```python
from build123d import *

# Parameters (mm, degrees)
BOSS_EXTRUDE1_DEPTH = 3.175
BOSS_EXTRUDE3_DEPTH = 152.4
BOSS_EXTRUDE4_DEPTH = 3.175
FILLET1_R           = 3.175
CHAMFER1_SIZE2      = 11.849261314
CHAMFER1_SIZE       = 3.175
SKETCH4_R           = 1.905
CUT_EXTRUDE1_DEPTH  = 158.75
CUT_EXTRUDE2_DEPTH  = 254


# Some blends are built 0.0001 mm under size
with BuildPart() as part:
    # Sketch1 → Boss-Extrude1 (new body)
    with BuildSketch(Plane(origin=(0, 0, 0), x_dir=(1, 0, 0), z_dir=(0, 1, 0))):
        Polygon((0, 0), (76.2, 0), (76.2, 63.5), (-17.014773719, 63.5), align=None)
    extrude(amount=BOSS_EXTRUDE1_DEPTH)

    # Sketch2 → Boss-Extrude3 (add)
    with BuildSketch(Plane(origin=(0, 3.175, 0), x_dir=(1, 0, 0), z_dir=(0, 1, 0))):
        Polygon((76.2, 0), (0, 0), (-17.014773719, 63.5), (-13.727771847, 63.5), (2.436263187, 3.175), (76.2, 3.175), align=None)
    extrude(amount=BOSS_EXTRUDE3_DEPTH)

    # Sketch3 → Boss-Extrude4 (add)
    with BuildSketch(Plane(origin=(0, 155.575, 0), x_dir=(1, 0, 0), z_dir=(0, 1, 0))):
        Polygon((-17.014773719, 63.5), (0, 0), (76.2, 0), (76.2, 63.5), align=None)
    extrude(amount=BOSS_EXTRUDE4_DEPTH)

    # Fillet1
    # the kernel refuses this fillet: 3.175 mm, written as the material it takes off along each edge
    with BuildSketch(Plane(origin=(2.436263187, 3.175, -3.175), x_dir=(-0.9659258262890689, 0, 0.2588190451025188), z_dir=(0, -1, 0))) as fillet1_piece_1_section:
        Polygon((0, 0), (FILLET1_R * 1.02, 0), (FILLET1_R * 1.02, -FILLET1_R * 0.782673527739), (FILLET1_R * 0.263995426005, -FILLET1_R * 0.985244342815), align=None)
    fillet1_piece_1 = extrude(amount=FILLET1_R * 1.02, mode=Mode.PRIVATE)
    fillet1_piece_1 = fillet1_piece_1 - Plane(origin=(2.436263187, 3.175, -3.175), x_dir=(0.6087614290087213, 0, -0.7933533402912346), z_dir=(0, -1, 0)) * Sphere(FILLET1_R, mode=Mode.PRIVATE)
    add(fillet1_piece_1, mode=Mode.SUBTRACT)
    with BuildSketch(Plane(origin=(2.436263187, 155.575, -3.175), x_dir=(0, 0, 1), z_dir=(0, 1, 0))) as fillet1_piece_2_section:
        Polygon((0, 0), (FILLET1_R * 1.02, 0), (FILLET1_R * 1.02, -FILLET1_R * 0.782673527739), (FILLET1_R * 0.263995426005, -FILLET1_R * 0.985244342815), align=None)
    fillet1_piece_2 = extrude(amount=FILLET1_R * 1.02, mode=Mode.PRIVATE)
    fillet1_piece_2 = fillet1_piece_2 - Plane(origin=(2.436263187, 155.575, -3.175), x_dir=(0.6087614290087213, 0, -0.7933533402912346), z_dir=(0, 1, 0)) * Sphere(FILLET1_R, mode=Mode.PRIVATE)
    add(fillet1_piece_2, mode=Mode.SUBTRACT)
    with BuildSketch(Plane(origin=(-17.014773719, 158.75, -63.5), x_dir=(1, 0, 0), z_dir=(0, -1, 0))) as fillet1_piece_3:
        with BuildLine():
            CenterArc((FILLET1_R * 1.30322537284, FILLET1_R), FILLET1_R, 165, 105)
            Line((FILLET1_R * 0.337299546552, FILLET1_R * 1.2588190451), (FILLET1_R * 0.317981030026, FILLET1_R * 1.263995426))
            Line((FILLET1_R * 0.317981030026, FILLET1_R * 1.263995426), (-FILLET1_R * 0.0260645074568, -FILLET1_R * 0.02))
            Line((-FILLET1_R * 0.0260645074568, -FILLET1_R * 0.02), (FILLET1_R * 1.30322537284, -FILLET1_R * 0.02))
            Line((FILLET1_R * 1.30322537284, -FILLET1_R * 0.02), (FILLET1_R * 1.30322537284, 0))
        make_face()
    extrude(amount=158.75, mode=Mode.SUBTRACT)
    with BuildSketch(Plane(origin=(2.436263187, 0, 0), x_dir=(0, 1, 0), z_dir=(1, 0, 0))) as fillet1_piece_4:
        with BuildLine():
            CenterArc((FILLET1_R, -FILLET1_R), FILLET1_R, 90, 90)
            Line((0, -FILLET1_R), (-FILLET1_R * 0.02, -FILLET1_R))
            Line((-FILLET1_R * 0.02, -FILLET1_R), (-FILLET1_R * 0.02, FILLET1_R * 0.02))
            Line((-FILLET1_R * 0.02, FILLET1_R * 0.02), (FILLET1_R, FILLET1_R * 0.02))
            Line((FILLET1_R, FILLET1_R * 0.02), (FILLET1_R, 0))
        make_face()
    extrude(amount=73.763736813, mode=Mode.SUBTRACT)
    with BuildSketch(Plane(origin=(-19.06914989, 0, -71.167036246), x_dir=(0.9659258262890688, 0, -0.25881904510251874), z_dir=(0.2588190451025188, 0, 0.9659258262890689))) as fillet1_piece_5_section:
        with BuildLine():
            CenterArc((FILLET1_R, FILLET1_R), FILLET1_R, 180, 90)
            Line((0, FILLET1_R), (-FILLET1_R * 0.02, FILLET1_R))
            Line((-FILLET1_R * 0.02, FILLET1_R), (-FILLET1_R * 0.02, -FILLET1_R * 0.02))
            Line((-FILLET1_R * 0.02, -FILLET1_R * 0.02), (FILLET1_R, -FILLET1_R * 0.02))
            Line((FILLET1_R, -FILLET1_R * 0.02), (FILLET1_R, 0))
        make_face()
    fillet1_piece_5 = extrude(amount=71.241274269, mode=Mode.PRIVATE)
    fillet1_piece_5 = split(fillet1_piece_5, bisect_by=Plane(origin=(-8.105416373, 0.719979608, -63.5), z_dir=(0, 0, 1)), keep=Keep.TOP, mode=Mode.PRIVATE)
    add(fillet1_piece_5, mode=Mode.SUBTRACT)
    with BuildSketch(Plane(origin=(0, 155.575, 0), x_dir=(1, 0, 0), z_dir=(0, -1, 0))) as fillet1_piece_6:
        with BuildLine():
            CenterArc((FILLET1_R * 0.767326987979, -FILLET1_R), FILLET1_R, 90, 75)
            Line((-FILLET1_R * 0.19859883831, -FILLET1_R * 0.741180954897), (-FILLET1_R * 0.217917354836, -FILLET1_R * 0.736004573995))
            Line((-FILLET1_R * 0.217917354836, -FILLET1_R * 0.736004573995), (-FILLET1_R * 0.0153465397596, FILLET1_R * 0.02))
            Line((-FILLET1_R * 0.0153465397596, FILLET1_R * 0.02), (FILLET1_R * 0.767326987979, FILLET1_R * 0.02))
            Line((FILLET1_R * 0.767326987979, FILLET1_R * 0.02), (FILLET1_R * 0.767326987979, 0))
        make_face()
    extrude(amount=152.4, mode=Mode.SUBTRACT)
    with BuildSketch(Plane(origin=(2.436263187, 158.75, 0), x_dir=(0, -1, 0), z_dir=(1, 0, 0))) as fillet1_piece_7:
        with BuildLine():
            CenterArc((FILLET1_R, FILLET1_R), FILLET1_R, 180, 90)
            Line((0, FILLET1_R), (-FILLET1_R * 0.02, FILLET1_R))
            Line((-FILLET1_R * 0.02, FILLET1_R), (-FILLET1_R * 0.02, -FILLET1_R * 0.02))
            Line((-FILLET1_R * 0.02, -FILLET1_R * 0.02), (FILLET1_R, -FILLET1_R * 0.02))
            Line((FILLET1_R, -FILLET1_R * 0.02), (FILLET1_R, 0))
        make_face()
    extrude(amount=73.763736813, mode=Mode.SUBTRACT)
    with BuildSketch(Plane(origin=(-19.06914989, 158.75, -71.167036246), x_dir=(0.9659258262890688, 0, -0.25881904510251874), z_dir=(0.2588190451025188, 0, 0.9659258262890689))) as fillet1_piece_8_section:
        with BuildLine():
            CenterArc((FILLET1_R, -FILLET1_R), FILLET1_R, 90, 90)
            Line((0, -FILLET1_R), (-FILLET1_R * 0.02, -FILLET1_R))
            Line((-FILLET1_R * 0.02, -FILLET1_R), (-FILLET1_R * 0.02, FILLET1_R * 0.02))
            Line((-FILLET1_R * 0.02, FILLET1_R * 0.02), (FILLET1_R, FILLET1_R * 0.02))
            Line((FILLET1_R, FILLET1_R * 0.02), (FILLET1_R, 0))
        make_face()
    fillet1_piece_8 = extrude(amount=71.241274269, mode=Mode.PRIVATE)
    fillet1_piece_8 = split(fillet1_piece_8, bisect_by=Plane(origin=(-8.105416373, 158.030020392, -63.5), z_dir=(0, 0, 1)), keep=Keep.TOP, mode=Mode.PRIVATE)
    add(fillet1_piece_8, mode=Mode.SUBTRACT)
    with BuildSketch(Plane(origin=(-17.014773719, 169.094351397, -63.5), x_dir=(1, 0, 0), z_dir=(0, -1, 0))) as fillet1_piece_9a_section:
        with BuildLine():
            CenterArc((FILLET1_R * 1.30322537284, FILLET1_R), FILLET1_R, 165, 105)
            Line((FILLET1_R * 0.337299546552, FILLET1_R * 1.2588190451), (FILLET1_R * 0.317981030026, FILLET1_R * 1.263995426))
            Line((FILLET1_R * 0.317981030026, FILLET1_R * 1.263995426), (-FILLET1_R * 0.0260645074568, -FILLET1_R * 0.02))
            Line((-FILLET1_R * 0.0260645074568, -FILLET1_R * 0.02), (FILLET1_R * 1.30322537284, -FILLET1_R * 0.02))
            Line((FILLET1_R * 1.30322537284, -FILLET1_R * 0.02), (FILLET1_R * 1.30322537284, 0))
        make_face()
    fillet1_piece_9a = extrude(amount=169.094351397, mode=Mode.PRIVATE)
    fillet1_piece_9a = split(fillet1_piece_9a, bisect_by=Plane(origin=(-15.793777483, 158.75, -62.563096636), z_dir=(0, 1, 0)), keep=Keep.TOP, mode=Mode.PRIVATE)
    with BuildSketch(Plane(origin=(-19.06914989, 158.75, -71.167036246), x_dir=(0.9659258262890688, 0, -0.25881904510251874), z_dir=(0.2588190451025188, 0, 0.9659258262890689))) as fillet1_piece_9b_section:
        with BuildLine():
            CenterArc((FILLET1_R, -FILLET1_R), FILLET1_R, 90, 90)
            Line((0, -FILLET1_R), (-FILLET1_R * 0.02, -FILLET1_R))
            Line((-FILLET1_R * 0.02, -FILLET1_R), (-FILLET1_R * 0.02, FILLET1_R * 0.02))
            Line((-FILLET1_R * 0.02, FILLET1_R * 0.02), (FILLET1_R, FILLET1_R * 0.02))
            Line((FILLET1_R, FILLET1_R * 0.02), (FILLET1_R, 0))
        make_face()
    fillet1_piece_9b = extrude(amount=71.241274269, mode=Mode.PRIVATE)
    fillet1_piece_9b = split(fillet1_piece_9b, bisect_by=Plane(origin=(-17.307274922, 158.04031756, -63.5), z_dir=(0, 0, -1)), keep=Keep.TOP, mode=Mode.PRIVATE)
    fillet1_piece_9 = fillet1_piece_9a & fillet1_piece_9b
    add(fillet1_piece_9, mode=Mode.SUBTRACT)
    with BuildSketch(Plane(origin=(-19.06914989, 0, -71.167036246), x_dir=(0.9659258262890688, 0, -0.25881904510251874), z_dir=(0.2588190451025188, 0, 0.9659258262890689))) as fillet1_piece_10a_section:
        with BuildLine():
            CenterArc((FILLET1_R, FILLET1_R), FILLET1_R, 180, 90)
            Line((0, FILLET1_R), (-FILLET1_R * 0.02, FILLET1_R))
            Line((-FILLET1_R * 0.02, FILLET1_R), (-FILLET1_R * 0.02, -FILLET1_R * 0.02))
            Line((-FILLET1_R * 0.02, -FILLET1_R * 0.02), (FILLET1_R, -FILLET1_R * 0.02))
            Line((FILLET1_R, -FILLET1_R * 0.02), (FILLET1_R, 0))
        make_face()
    fillet1_piece_10a = extrude(amount=71.241274269, mode=Mode.PRIVATE)
    fillet1_piece_10a = split(fillet1_piece_10a, bisect_by=Plane(origin=(-17.307274922, 0.70968244, -63.5), z_dir=(0, 0, -1)), keep=Keep.TOP, mode=Mode.PRIVATE)
    with BuildSketch(Plane(origin=(-17.014773719, 158.75, -63.5), x_dir=(1, 0, 0), z_dir=(0, -1, 0))) as fillet1_piece_10b_section:
        with BuildLine():
            CenterArc((FILLET1_R * 1.30322537284, FILLET1_R), FILLET1_R, 165, 105)
            Line((FILLET1_R * 0.337299546552, FILLET1_R * 1.2588190451), (FILLET1_R * 0.317981030026, FILLET1_R * 1.263995426))
            Line((FILLET1_R * 0.317981030026, FILLET1_R * 1.263995426), (-FILLET1_R * 0.0260645074568, -FILLET1_R * 0.02))
            Line((-FILLET1_R * 0.0260645074568, -FILLET1_R * 0.02), (FILLET1_R * 1.30322537284, -FILLET1_R * 0.02))
            Line((FILLET1_R * 1.30322537284, -FILLET1_R * 0.02), (FILLET1_R * 1.30322537284, 0))
        make_face()
    fillet1_piece_10b = extrude(amount=169.094351397, mode=Mode.PRIVATE)
    fillet1_piece_10b = split(fillet1_piece_10b, bisect_by=Plane(origin=(-15.793777483, 0, -62.563096636), z_dir=(0, -1, 0)), keep=Keep.TOP, mode=Mode.PRIVATE)
    fillet1_piece_10 = fillet1_piece_10a & fillet1_piece_10b
    add(fillet1_piece_10, mode=Mode.SUBTRACT)

    # Chamfer1
    chamfer1_edges = [part.edges().sort_by_distance(p)[0] for p in [
        (76.2, 79.375, -3.175),
    ]]
    chamfer1_side = [part.faces().sort_by_distance(p)[0] for p in [
        (76.2, 79.375, -3.1115),
    ]]
    chamfer(chamfer1_edges, length=CHAMFER1_SIZE - 0.0001, length2=CHAMFER1_SIZE2 - 0.0001, reference=chamfer1_side[0])  # a hair under: the kernel refuses the full size

    # Sketch4 → Cut-Extrude1 (cut)
    with BuildSketch(Plane.XZ):
        with Locations(Location((6.35, -12.7, 0), (0, 0, 270))):
            Circle(SKETCH4_R)
    extrude(amount=-CUT_EXTRUDE1_DEPTH, mode=Mode.SUBTRACT)

    # Sketch6 → Cut-Extrude2 (cut)
    with BuildSketch(Plane(origin=(0, 158.75, 0), x_dir=(1, 0, 0), z_dir=(0, 1, 0))):
        Polygon((-13.698783629, 63.391814498), (76.2, 0), (76.2, 63.5), (-15.882639691, 64.0756894), align=None)
    extrude(amount=-CUT_EXTRUDE2_DEPTH, mode=Mode.SUBTRACT)


solid = part.part
```
The model under review builds one solid part; all positions refer to its coordinate system, in mm. A direction names the side the tool comes from. Round coordinates to 2 decimals unless told otherwise and drop trailing zeros. Order: outer loops, then holes, each group sorted by start corner. A loop starts at its lowest first (then second) coordinate and runs counter-clockwise, first axis right, second up.
(1) Take a section at B-B, the plane y = 80. State the section outline as (x, z) points (3 decimals), plus the area to 3 significant figures.
Working result:
outline: (-15.944, -59.503) arc R3.175 ccw to (-13.699, -63.392) - (2.436, -3.175) - (64.351, -3.175) - (76.2, 0) - (2.436, 0) arc R3.175 ccw to (-0.631, -2.353) - close
area: 418 mm2
(2) Take a section at D-D, the plane z = -12.7. Count the separate pieces of the cut face and the enclosed holes in it, plus the area to 3 significant figures.
Working result:
separate pieces: 3
enclosed holes: 0
area: 863 mm2
(3) Take a section at A-A, the plane x = 6.35. State the section outline as (y, z) points (3 decimals).
Working result:
outline: (0, -49.254) - (3.175, -49.254) - (3.175, -14.605) - (0, -14.605) - close; (0, -10.795) - (3.175, -10.795) - (3.175, -3.175) - (155.575, -3.175) - (155.575, -10.795) - (158.75, -10.795) - (158.75, -3.175) arc R3.175 ccw to (155.575, 0) - (3.175, 0) arc R3.175 ccw to (0, -3.175) - close; (155.575, -49.254) - (158.75, -49.254) - (158.75, -14.605) - (155.575, -14.605) - close
(4) Wall thickness on L1, parallel to Y at x = 32.5, z = -19 (3 decimals); L2, parallel to Z at x = 48, y = 47 (3 decimals); L3, parallel to Z at x = 6, y = 1: over which ranges is each line inside the solid? List them lowest first.
Working result:
L1: y = 0 to 3.175, 155.575 to 158.75
L2: z = -3.175 to 0
L3: z = -49.5 to -14.57, -10.83 to -0.86
(5) Mouldability with a two-part tool opening along Z and no side actions: class faces 1 (the face through (-7.889, 157.845, -33.13)), 2 (the face through (5.62, 157.14, -14.46)), 3 (the face through (30.62, 157.18, -32.14)) as released by +Z, released by -Z, zero draft, split by the parting line, or undercut.
Working result:
face 1: released by +Z
face 2: undercut
face 3: released by -Z
(6) For P1, Ø3.5, axis at x = 6.35, z = -12.7, coming from the +Y side; P2, Ø12, axis at y = 26.5, z = -31, coming from the +X side; P3, Ø4, axis at x = 49, y = 41, coming from the -Z side (3 decimals); P4, Ø10, axis at y = 125, z = -35.5, coming from the -X side, all flat-tipped, find the tip position at first contact; note any pin that passes through.
Working result:
P1: passes through
P2: stops at x = -3.41
P3: stops at z = -3.175
P4: stops at x = -10.85
(7) Tool access review of faces 4 (the face through (-15.644, 80.486, -61.882)), 5 (the face through (33, 78, -3.175)): name each direction out of +Z, -Z, +X, -X, +Y, -Y from which nothing blocks a thin tool from reaching the whole face with its end or side.
Working result:
face 4: -X, +Y, -Y
face 5: -Z, +X
(8) Take a section at C-C, the plane x = 24.5. State the section outline as (y, z) points (3 decimals).
Working result:
outline: (0, -36.456) - (3.175, -36.456) - (3.175, -3.175) - (155.575, -3.175) - (155.575, -36.456) - (158.75, -36.456) - (158.75, -3.175) arc R3.175 ccw to (155.575, 0) - (3.175, 0) arc R3.175 ccw to (0, -3.175) - close
